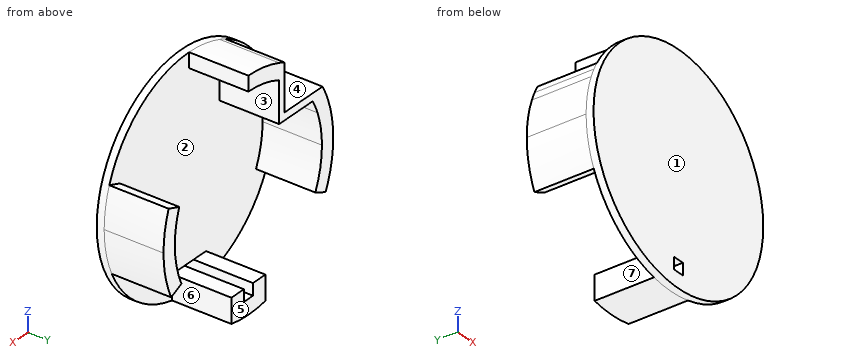
```python
from build123d import *

# Parameters (mm, degrees)
SKETCH1_R           = 75
BOSS_EXTRUDE1_DEPTH = 5
CUT_EXTRUDE1_DEPTH  = 10
BOSS_EXTRUDE3_DEPTH = 40


with BuildPart() as part:
    # Sketch1 → Boss-Extrude1 (new body)
    with BuildSketch(Plane(origin=(0, 0, 0), x_dir=(1, 0, 0), z_dir=(0, 1, 0))):
        with Locations((-5.935816789, 0)):
            Circle(SKETCH1_R)
    extrude(amount=BOSS_EXTRUDE1_DEPTH)

    # Sketch2 → Cut-Extrude1 (cut)
    with BuildSketch(Plane(origin=(0, 5, 0), x_dir=(1, 0, 0), z_dir=(0, 1, 0))):
        with BuildLine():
            Line((-1.948906052, 56.999998596), (-1.948906052, 64.87761203))
            ThreePointArc((-1.948906052, 64.87761203), (-5.948930907, 64.999998677), (-9.948906052, 64.875997985))
            Line((-9.948906052, 64.875997985), (-9.948906052, 56.999998596))
            Line((-9.948906052, 56.999998596), (-1.948906052, 56.999998596))
        make_face()
    extrude(amount=-CUT_EXTRUDE1_DEPTH, mode=Mode.SUBTRACT)

    # Sketch2_5 → Boss-Extrude3 (add)
    with BuildSketch(Plane(origin=(0, 5, 0), x_dir=(1, 0, 0), z_dir=(0, 1, 0))):
        with BuildLine():
            ThreePointArc((53.238004246, 26.89719138), (57.590942798, 13.760480237), (59.064183211, 0))
            Line((59.064183211, 0), (69.064183211, 0))
            ThreePointArc((69.064183211, 0), (67.364290427, 15.877477197), (62.34166902, 31.035220823))
            Line((62.34166902, 31.035220823), (53.238004246, 26.89719138))
        make_face()
        with BuildLine():
            ThreePointArc((59.064183211, 0), (58.078350448, -11.277694484), (55.150755737, -22.213299101))
            Line((55.150755737, -22.213299101), (64.548689972, -25.630729732))
            ThreePointArc((64.548689972, -25.630729732), (67.926683869, -13.012724405), (69.064183211, 0))
            Line((69.064183211, 0), (59.064183211, 0))
        make_face()
        with BuildLine():
            Line((-5.935816789, -75), (-5.935816789, -65))
            ThreePointArc((-5.935816789, -65), (-19.824804959, -63.49878745), (-33.072244718, -59.064492542))
            Line((-33.072244718, -59.064492542), (-33.072244718, -69.918626126))
            ThreePointArc((-33.072244718, -69.918626126), (-19.739856788, -73.71871187), (-5.935816789, -75))
        make_face()
        with BuildLine():
            Line((-33.072244718, -69.918626126), (-33.072244718, -59.064492542))
            ThreePointArc((-33.072244718, -59.064492542), (-35.599970508, -57.836303341), (-38.072244718, -56.5))
            Line((-38.072244718, -56.5), (-38.072244718, -67.766141988))
            ThreePointArc((-38.072244718, -67.766141988), (-35.591780057, -68.887762648), (-33.072244718, -69.918626126))
        make_face()
        with BuildLine():
            Line((-33.072244718, -59.064492542), (-33.072244718, -36.5))
            Line((-33.072244718, -36.5), (-38.072244718, -36.5))
            Line((-38.072244718, -36.5), (-38.072244718, -56.5))
            ThreePointArc((-38.072244718, -56.5), (-35.599970508, -57.836303341), (-33.072244718, -59.064492542))
        make_face()
        with BuildLine():
            Line((-38.072244718, -36.5), (-33.072244718, -36.5))
            Line((-33.072244718, -36.5), (-33.072244718, -31.5))
            Line((-33.072244718, -31.5), (-62.793094248, -31.5))
            ThreePointArc((-62.793094248, -31.5), (-61.313061115, -34.034700099), (-59.720108176, -36.5))
            Line((-59.720108176, -36.5), (-38.072244718, -36.5))
        make_face()
        with BuildLine():
            ThreePointArc((-59.720108176, -36.5), (-61.313061115, -34.034700099), (-62.793094248, -31.5))
            Line((-62.793094248, -31.5), (-74.000124617, -31.5))
            ThreePointArc((-74.000124617, -31.5), (-72.774282177, -34.023808497), (-71.454897979, -36.5))
            Line((-71.454897979, -36.5), (-59.720108176, -36.5))
        make_face()
        with BuildLine():
            Line((-74.000124617, -31.5), (-62.793094248, -31.5))
            ThreePointArc((-62.793094248, -31.5), (-65.090264135, -26.939772814), (-67.022389316, -22.213299101))
            Line((-67.022389316, -22.213299101), (-76.420323551, -25.630729732))
            ThreePointArc((-76.420323551, -25.630729732), (-75.272355421, -28.590984779), (-74.000124617, -31.5))
        make_face()
        with BuildLine():
            ThreePointArc((-67.022389316, -22.213299101), (-69.949984027, -11.277694484), (-70.935816789, 0))
            Line((-70.935816789, 0), (-80.935816789, 0))
            ThreePointArc((-80.935816789, 0), (-79.798317448, -13.012724405), (-76.420323551, -25.630729732))
            Line((-76.420323551, -25.630729732), (-67.022389316, -22.213299101))
        make_face()
        with BuildLine():
            Line((-80.935816789, 0), (-70.935816789, 0))
            ThreePointArc((-70.935816789, 0), (-69.462576376, 13.760480237), (-65.109637824, 26.89719138))
            Line((-65.109637824, 26.89719138), (-74.213302599, 31.035220823))
            ThreePointArc((-74.213302599, 31.035220823), (-79.235924005, 15.877477197), (-80.935816789, 0))
        make_face()
        with BuildLine():
            ThreePointArc((-9.948906052, 64.875997985), (-15.483905038, 64.294898793), (-20.948906052, 63.242447382))
            Line((-20.948906052, 63.242447382), (-20.948906052, 56.999998596))
            Line((-20.948906052, 56.999998596), (-9.948906052, 56.999998596))
            Line((-9.948906052, 56.999998596), (-9.948906052, 64.875997985))
        make_face()
        with BuildLine():
            ThreePointArc((-1.948906052, 64.87761203), (3.585992369, 64.29879587), (9.051093948, 63.248656164))
            Line((9.051093948, 63.248656164), (9.051093948, 73.487362904))
            ThreePointArc((9.051093948, 73.487362904), (-5.949175962, 74.99999881), (-20.948906052, 73.482019235))
            Line((-20.948906052, 73.482019235), (-20.948906052, 63.242447382))
            ThreePointArc((-20.948906052, 63.242447382), (-15.483905038, 64.294898793), (-9.948906052, 64.875997985))
            ThreePointArc((-9.948906052, 64.875997985), (-5.948930907, 64.999998677), (-1.948906052, 64.87761203))
        make_face()
        with BuildLine():
            Line((9.051093948, 56.999998596), (9.051093948, 63.248656164))
            ThreePointArc((9.051093948, 63.248656164), (3.585992369, 64.29879587), (-1.948906052, 64.87761203))
            Line((-1.948906052, 64.87761203), (-1.948906052, 56.999998596))
            Line((-1.948906052, 56.999998596), (9.051093948, 56.999998596))
        make_face()
    extrude(amount=BOSS_EXTRUDE3_DEPTH)


solid = part.part
```
Here's how the part is built. I have some questions about the finished solid (model axes, mm). Face numbers are marked on the shaded views. A direction names the side the tool comes from. Round coordinates to 2 decimals unless told otherwise and drop trailing zeros. Loops run counter-clockwise (first coordinate to the right, second up) from the corner with the lowest first, then second, coordinate; pieces in that order, holes last. Notation, with made-up numbers: (5.25, 37) -> (37.25, 37) arc R23 cw to (37.25, 60) -> close; hole circle Ø4 at (66.5, 48.25). An arc over 180 degrees is marked (long way). Answer as CSV lines item,"result".
1. If we section it at B-B on z = 56: Please give me the cut outline in (x, y), plus the area to 3 significant figures.
Final values:
outline,"(-55.83, 0) -> (43.95, 0) -> (43.95, 5) -> (-33.07, 5) -> (-33.07, 45) -> (-38.07, 45) -> (-38.07, 5) -> (-55.83, 5) -> close"
area,"699 mm^2"
2. Thinking about a two-plate mould opening in X: for the marked faces 1, 2 and 3, which applies, released by +X, released by -X, zero draft, split by the parting line, or undercut?
Final values:
face 1,"zero draft"
face 2,"undercut"
face 3,"released by +X"
3. If we section it at D-D on x = -23.5: Please give me the cut outline in (y, z).
Final values:
outline,"(0, -72.91) -> (5, -72.91) -> (5, 62.58) -> (45, 62.58) -> (45, 72.91) -> (0, 72.91) -> close"
4. If we section it at A-A on y = 27.5: Please give me the cut outline in (x, z), plus the area to 3 significant figures.
Final values:
outline,"(-74.21, -31.04) -> (-65.11, -26.9) arc R65 cw to (-62.79, 31.5) -> (-33.07, 31.5) -> (-33.07, 59.06) arc R65 cw to (-5.94, 65) -> (-5.94, 75) arc R75 ccw to (-38.07, 67.77) -> (-38.07, 36.5) -> (-71.45, 36.5) arc R75 ccw to start; (-20.95, -73.48) arc R75 ccw to (9.05, -73.49) -> (9.05, -57) -> (-1.95, -57) -> (-1.95, -64.88) arc R65 cw to (-9.95, -64.88) -> (-9.95, -57) -> (-20.95, -57) -> close; (53.24, -26.9) -> (62.34, -31.04) arc R75 ccw to (64.55, 25.63) -> (55.15, 22.21) arc R65 cw to start"
area,"2,270 mm^2"
5. For pin 1 (12 mm diameter, centred on x = 6, y = 19, fed in from +Z); pin 2 (1.5 mm diameter, centred on x = -58, z = 10.5, fed in from +Y); pin 3 (6 mm diameter, centred on x = -57.5, y = 12, fed in from +Z), each with a flat end and sliding along its axis, tell me the tip position at first contact or that it passes through.
Final values:
pin 1,"stops at z = -57"
pin 2,"stops at y = 5"
pin 3,"stops at z = 36.5"
6. If we section it at C-C on x = -61: Please give me the cut outline in (y, z).
Final values:
outline,"(0, -50.92) -> (5, -50.92) -> (5, 31.5) -> (45, 31.5) -> (45, 36.5) -> (5, 36.5) -> (5, 50.92) -> (0, 50.92) -> close"
7. Which directions (+Z, -Z, +X, -X, +Y, -Y) give clear straight access to the entire face, cutting with the end or side of a thin tool? Please do the marked faces 4, 5, 6 and 7.
Final values:
face 4,"+Z, -X, +Y"
face 5,"+Z, -Z, +X, -X, +Y"
face 6,"+Z, -Z, +X, +Y"
face 7,"-Z, -X, +Y"
8. If I drill on L1, parallel to Y at x = 36.5, z = -17; L2, parallel to Z at x = -60, y = 41.5; L3, parallel to Z at x = -10.5, y = 30, over which ranges is the centre line in solid material (lowest first)?
Final values:
L1,"y = 0 to 5"
L2,"z = 31.5 to 36.5"
L3,"z = -74.86 to -57, 64.84 to 74.86"
